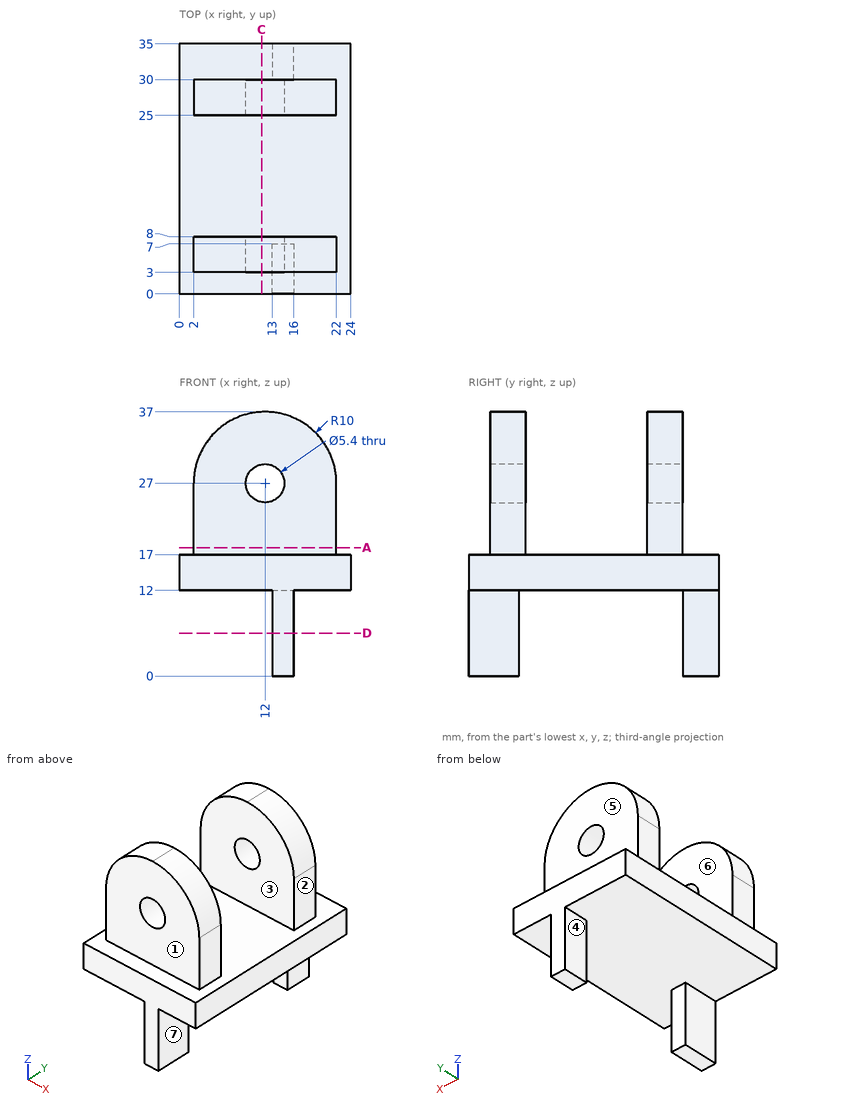
Drawing for the job (mm, zero at the part's lowest x, y, z). A direction names the side the tool comes from. Coordinates: 2 decimals unless noted, no trailing zeros. Write each loop counter-clockwise with the first axis right and the second up, starting at its lowest first coordinate (ties: lowest second). Pieces come first, ordered by that corner, then holes. Notation, with made-up numbers: (20, -15) -> (52, -15) arc R21 cw to (52, -2) -> close; hole circle Ø6 at (41, -0.75). An arc over 180 degrees is marked (long way). One line per item, written item: value. Start each with the question number.
1) Slice it at A-A on z = 18. Write the cut outline in (x, y), then the cut area to 3 significant figures.
2) Slice it at C-C on x = 11.5. Write the cut outline in (y, z).
3) Slice it at D-D on z = 6. Write the cut outline in (x, y).
4) Probe probe 1 along X at (y, z) = (26.6, 27); probe 2 along Z at (x, y) = (12, 27.9); probe 3 along Y at (x, z) = (19.25, 31). List the from-to ranges inside material, lowest first.
5) Flat gauge pins, fed straight in: pin 1 Ø1 at (y, z) = (30, 11) entering from +X; pin 2 Ø2.5 at (y, z) = (6, 20.5) entering from -X; pin 3 Ø5.5 at (y, z) = (5, 24.5) entering from +X. Where does each tip first touch, or does it go through?
6) Which spindle directions (+Z, -Z, +X, -X, +Y, -Y) get a long thin tool onto all of the face, cutting with end or side? Do the marked faces 4, 5, 6 and 7. Say none if no direction does.
7) Pull direction Y, two halves, no side cores. Call the marked faces 1, 2 and 3: +Y half, -Y half, draft (parallel to the pull), parting line (faces both ways), or undercut.
Answers follow:
1. outline: (2, 3) -> (22, 3) -> (22, 8) -> (2, 8) -> close; (2, 25) -> (22, 25) -> (22, 30) -> (2, 30) -> close
1. area: 200 mm2
2. outline: (0, 12) -> (35, 12) -> (35, 17) -> (30, 17) -> (30, 24.35) -> (25, 24.35) -> (25, 17) -> (8, 17) -> (8, 24.35) -> (3, 24.35) -> (3, 17) -> (0, 17) -> close; (3, 29.65) -> (8, 29.65) -> (8, 36.99) -> (3, 36.99) -> close; (25, 29.65) -> (30, 29.65) -> (30, 36.99) -> (25, 36.99) -> close
3. outline: (13, 0) -> (16, 0) -> (16, 7) -> (13, 7) -> close; (13, 30) -> (16, 30) -> (16, 35) -> (13, 35) -> close
4. probe 1: 2 to 9.3, 14.7 to 22
4. probe 2: 12 to 24.3, 29.7 to 37
4. probe 3: 3 to 8, 25 to 30
5. pin 1: x = 16
5. pin 2: x = 2
5. pin 3: x = 22
6. face 4: -Z, -X, +Y, -Y
6. face 5: +Z, +X, -X, +Y
6. face 6: +Z, +X, -X
6. face 7: -Z, +X, +Y, -Y
7. face 1: -Y half
7. face 2: draft
7. face 3: undercut
